from build123d import *

# Parameters (mm, degrees)
F2_SIZE  = 0.5
F4_DEPTH = 3


with BuildPart() as f1:
    # F0 (on Front) → F1 (revolve)
    with BuildSketch(Plane.XZ):
        Polygon((-4.1, 0), (0, 0), (0, 5), (-11.1, 5), (-11.1, 4), (-5.1, 4), (-5.1, 3), (-4.1, 3), align=None)
    revolve(axis=Axis((0, 0, 2.5), (0, 0, -1)))

    # F2
    f2_edges = [f1.edges().sort_by_distance(p)[0] for p in [
        (11.1, 0, 5),
    ]]
    chamfer(f2_edges, length=F2_SIZE)

    # F3 (on face) → F4 (cut)
    with BuildSketch(Plane(origin=(0, 0, 0), x_dir=(1, 0, 0), z_dir=(0, 0, -1))):
        with BuildLine():
            ThreePointArc((2.40992, 3.31697), (1.26697, 3.899332), (0, 4.1))
            Line((0, 4.1), (2.40992, 3.31697))
        make_face()
        with BuildLine():
            ThreePointArc((3.899332, 1.26697), (3.31697, 2.40992), (2.40992, 3.31697))
            Line((2.40992, 3.31697), (3.899332, 1.26697))
        make_face()
        with BuildLine():
            ThreePointArc((4.1, 0), (4.049522, 0.641381), (3.899332, 1.26697))
            Line((3.899332, 1.26697), (3.899332, -1.26697))
            ThreePointArc((3.899332, -1.26697), (4.049522, -0.641381), (4.1, 0))
        make_face()
        with BuildLine():
            ThreePointArc((2.40992, -3.31697), (3.31697, -2.40992), (3.899332, -1.26697))
            Line((3.899332, -1.26697), (2.40992, -3.31697))
        make_face()
        with BuildLine():
            ThreePointArc((0, -4.1), (1.26697, -3.899332), (2.40992, -3.31697))
            Line((2.40992, -3.31697), (0, -4.1))
        make_face()
        with BuildLine():
            Line((0, -4.1), (-2.40992, -3.31697))
            ThreePointArc((-2.40992, -3.31697), (-1.26697, -3.899332), (0, -4.1))
        make_face()
        with BuildLine():
            Line((-2.40992, -3.31697), (-3.899332, -1.26697))
            ThreePointArc((-3.899332, -1.26697), (-3.31697, -2.40992), (-2.40992, -3.31697))
        make_face()
        with BuildLine():
            Line((-3.899332, -1.26697), (-3.899332, 1.26697))
            ThreePointArc((-3.899332, 1.26697), (-4.1, 0), (-3.899332, -1.26697))
        make_face()
        with BuildLine():
            Line((-3.899332, 1.26697), (-2.40992, 3.31697))
            ThreePointArc((-2.40992, 3.31697), (-3.31697, 2.40992), (-3.899332, 1.26697))
        make_face()
        with BuildLine():
            Line((-2.40992, 3.31697), (0, 4.1))
            ThreePointArc((0, 4.1), (-1.26697, 3.899332), (-2.40992, 3.31697))
        make_face()
    extrude(amount=-F4_DEPTH, mode=Mode.SUBTRACT)


solid = f1.part
Build history of the part. All positions in model axes, mm. A direction names the side the tool comes from. Give positions to 0.01 mm unless a question says otherwise; leave off trailing zeros. Write each loop counter-clockwise with the first axis right and the second up, starting at its lowest first coordinate (ties: lowest second). Pieces come first, ordered by that corner, then holes. Notation, with made-up numbers: (-6, 35.25) - (45, 35.25) arc R17 ccw to (45, 43.25) - close; hole circle Ø4 at (-1.75, 8.25). An arc over 180 degrees is marked (long way). Use one line per item in the form item = value. Start each with the question number.
1. Band-saw the part on A-A on y = 0. Write the cut outline in (x, z).
2. 3-axis set-ups, long thin cutter, end or side, ignore diameter. For faces 1 (the face through (-2.4, -4.5, 3.5)), 2 (the face through (3.899, 0, 1)), 3 (the face through (-3.165, -2.278, 1.479)), 4 (the face through (3.14, -2.31, 1.48)), 5 (the face through (-3.14, 2.31, 1.48)): which of +Z, -Z, +X, -X, +Y, -Y reach the whole face in a straight line?
3. Drop flat-ended pins along their axis: pin 1 Ø2 at (y, z) = (-0.5, 1.5) entering from +X; pin 2 Ø1.5 at (y, z) = (1, 2.5) entering from +X; pin 3 Ø3 at (y, z) = (0.5, 2) entering from -X. Give the stop position or say it passes through.
4. Probe line 1 (Z direction, x = 8.25, y = 6); line 2 (X direction, y = 0, z = 0.3); line 3 (Z direction, x = -0.5, y = 4.5). List the from-to ranges inside material, lowest first. Write a range as [from, to].
Conclusion:
q1.outline = (-11.1, 4) - (-5.1, 4) - (-5.1, 3) - (-3.9, 3) - (-3.9, 0) - (3.9, 0) - (3.9, 3) - (5.1, 3) - (5.1, 4) - (11.1, 4) - (11.1, 4.5) - (10.6, 5) - (-10.6, 5) - (-11.1, 4.5) - close
q2.face_1 = -Z
q2.face_2 = -Z, +X, +Y, -Y
q2.face_3 = -Z, -X, -Y
q2.face_4 = -Z, +X, -Y
q2.face_5 = -Z, -X, +Y
q3.pin_1 = 3.9
q3.pin_2 = 5.08
q3.pin_3 = -5.1
q4.line_1 = [4, 5]
q4.line_2 = [-3.9, 3.9]
q4.line_3 = [3, 5]
